Could you check a few things on this model? Use its own coordinates, in mm. A direction names the side the tool comes from. Coordinates: 2 decimals unless noted, no trailing zeros. Order: outer loops, then holes, each group sorted by start corner. A loop starts at its lowest first (then second) coordinate and runs counter-clockwise, first axis right, second up. Notation, with made-up numbers: (20, 57) -> (39, 57) arc R32 ccw to (39, 85) -> close; hole circle Ø4 at (3.5, -24). An arc over 180 degrees is marked (long way). Return JSON: item names as keys, results as strings. Group by question number.
Autodesk Inventor part; units mm, degrees
ref_plane "YZ Plane" through (0, 0, 0) normal (1, 0, 0) x (0, 1, 0)
ref_plane "XZ Plane" through (0, 0, 0) normal (0, 1, 0) x (-1, 0, 0)
ref_plane "XY Plane" through (0, 0, 0) normal (0, 0, 1) x (1, 0, 0)
sketch "Sketch1" plane through (0, 0, 0) normal (0, 1, 0) x (-1, 0, 0)
  line L0 (0, 0) -> (12, 0)
  line L1 (12, 0) -> (12, -144.6)
  line L2 (12, -144.6) -> (0, -144.6)
  line L3 (0, -144.6) -> (0, 0)
  line L4 (0, 0) -> (3, 0)
  line L5 (3, 0) -> (3, -4)
  line L6 (3, -4) -> (0, -4)
  line L7 (0, -4) -> (0, 0)
  line L8 (3, -4) -> (9, -4)
  circle A0 centre (9, -4) radius 1.5
  circle A1 centre (3, -4) radius 1.5
  line L9 (12, -144.6) -> (9, -144.6)
  line L10 (9, -144.6) -> (9, -140.6)
  line L11 (9, -140.6) -> (12, -140.6)
  line L12 (12, -140.6) -> (12, -144.6)
  line L13 (9, -140.6) -> (3, -140.6)
  circle A2 centre (9, -140.6) radius 1.5
  circle A3 centre (3, -140.6) radius 1.5
  dimension "d0" = 12
  dimension "d1" = 144.6
  dimension "d2" = 3
  dimension "d3" = 4
  dimension "d4" = 6
  dimension "d5" = 3
  dimension "d6" = 3
  dimension "d7" = 3
  dimension "d8" = 4
  dimension "d9" = 6
  dimension "d10" = 3
  dimension "d11" = 3
extrude "Extrusion1" add sketch "Sketch1" along normal blind 3 contours L0 L5 A1 L6 L3 | L0 L1 L11 A2 L10 L2 L3 L6 A1 L5 | L1 L2 L10 A2 L11
sketch "Sketch2" plane through (0, 3, 0) normal (0, 1, 0) x (1, 0, 0)
  line L0 (-12, 0) -> (0, 0)
  line L1 (-6, 0) -> (-6, 144.6) construction
  line L2 (0, 144.6) -> (-12, 144.6)
  line L3 (-4.5, 0) -> (-4.5, 144.6)
  line L4 (-7.5, 144.6) -> (-7.5, 0)
  arc A0 (-7.5, 0) -> (-4.5, 0) centre (-6, 0) ccw
  arc A1 (-4.5, 144.6) -> (-7.5, 144.6) centre (-6, 144.6) ccw
  line L5 (0, 0) -> (0, 144.6)
  line L6 (-12, 0) -> (0, 0)
  line L7 (0, 0) -> (0, 8)
  line L8 (0, 8) -> (-12, 8)
  line L9 (-12, 8) -> (-12, 0)
  line L10 (-12, 144.6) -> (0, 144.6)
  line L11 (0, 144.6) -> (0, 136.6)
  line L12 (0, 136.6) -> (-12, 136.6)
  line L13 (-12, 136.6) -> (-12, 144.6)
  point P0 (-6, 72.3)
  point P1 (-4.5, 136.6)
  point P2 (-7.5, 136.6)
  point P3 (-7.5, 8)
  point P4 (-4.5, 8)
  dimension "d14" = 3
  dimension "d15" = 8
  dimension "d16" = 8
extrude "Extrusion2" add sketch "Sketch2" along normal blind 3 contours L4 L12 L3 L8
fillet "Fillet1" radius 3 2 edges at (-6, 6, -8) (-6, 6, -136.6)
fillet "Fillet2" radius 3 4 edges at (0, 1.5, 0) (-12, 1.5, 0) (-12, 1.5, -144.6) (0, 1.5, -144.6)
fillet "Fillet3" radius 1.5 6 edges at (-7.5, 5.1215, -8.8785) (-7.5, 5.1215, -135.7215) (-7.5, 6, -72.3) (-4.5, 5.1215, -135.7215) (-4.5, 5.1215, -8.8785) (-4.5, 6, -72.3)
sketch "Sketch3" plane through (0, 3, 0) normal (0, 1, 0) x (1, 0, 0)
  line L0 (-12, 141.6) -> (-12, 3)
  line L1 (-12, 72.3) -> (-6, 72.3)
  line L2 (-9, 42.3) -> (-3, 42.3)
  line L3 (-3, 42.3) -> (-3, 102.3)
  line L4 (-3, 102.3) -> (-9, 102.3)
  line L5 (-9, 102.3) -> (-9, 42.3)
  line L6 (-9, 42.3) -> (-3, 102.3) construction
  line L7 (-3, 42.3) -> (-9, 102.3) construction
  line L8 (-9, 32.3) -> (-3, 32.3)
  line L9 (-3, 32.3) -> (-3, 112.3)
  line L10 (-3, 112.3) -> (-9, 112.3)
  line L11 (-9, 112.3) -> (-9, 32.3)
  line L12 (-9, 32.3) -> (-3, 112.3) construction
  line L13 (-3, 32.3) -> (-9, 112.3) construction
  line L14 (-9, 112.3) -> (-3, 112.3) construction
  line L15 (-9, 109.3) -> (-3, 109.3)
  line L16 (-3, 115.3) -> (-9, 115.3)
  arc A0 (-9, 115.3) -> (-9, 109.3) centre (-9, 112.3) ccw
  arc A1 (-3, 109.3) -> (-3, 115.3) centre (-3, 112.3) ccw
  circle A2 centre (-9, 112.3) radius 1.5
  circle A3 centre (-3, 112.3) radius 1.5
  circle A4 centre (-9, 102.3) radius 1.5
  circle A5 centre (-3, 102.3) radius 1.5
  line L17 (-9, 102.3) -> (-3, 102.3) construction
  line L18 (-9, 99.3) -> (-3, 99.3)
  line L19 (-3, 105.3) -> (-9, 105.3)
  arc A6 (-9, 105.3) -> (-9, 99.3) centre (-9, 102.3) ccw
  arc A7 (-3, 99.3) -> (-3, 105.3) centre (-3, 102.3) ccw
  line L20 (-3, 32.3) -> (-9, 32.3)
  line L21 (-3, 42.3) -> (-9, 42.3)
  line L22 (-9, 42.3) -> (-3, 42.3) construction
  line L23 (-9, 39.3) -> (-3, 39.3)
  line L24 (-3, 45.3) -> (-9, 45.3)
  arc A8 (-9, 45.3) -> (-9, 39.3) centre (-9, 42.3) ccw
  arc A9 (-3, 39.3) -> (-3, 45.3) centre (-3, 42.3) ccw
  circle A10 centre (-9, 42.3) radius 1.5
  circle A11 centre (-3, 42.3) radius 1.5
  circle A12 centre (-9, 32.3) radius 1.5
  circle A13 centre (-3, 32.3) radius 1.5
  line L25 (-9, 32.3) -> (-3, 32.3) construction
  line L26 (-9, 29.3) -> (-3, 29.3)
  line L27 (-3, 35.3) -> (-9, 35.3)
  arc A14 (-9, 35.3) -> (-9, 29.3) centre (-9, 32.3) ccw
  arc A15 (-3, 29.3) -> (-3, 35.3) centre (-3, 32.3) ccw
  point P0 (0, 0)
  point P1 (-6, 112.3)
  point P2 (-6, 102.3)
  point P3 (-6, 42.3)
  point P4 (-6, 32.3)
  dimension "d22" = 6
  dimension "d23" = 6
  dimension "d24" = 60
  dimension "d25" = 6
  dimension "d26" = 80
  dimension "d27" = 6
  dimension "d28" = 3
  dimension "d29" = 3
  dimension "d30" = 3
  dimension "d31" = 3
  dimension "d32" = 6
  dimension "d33" = 6
  dimension "d34" = 6
  dimension "d35" = 6
  dimension "d36" = 3
  dimension "d37" = 3
  dimension "d38" = 3
  dimension "d39" = 3
  dimension "d40" = 6
extrude "Extrusion3" cut sketch "Sketch3" along normal blind 3 contours A0 L16 A1 L9 A3 L10 A2 L11 | A6 L11 A4 L5 | L11 A2 L10 A3 L9 L15 | L19 L9 A5 L4 A4 L11 | L5 A4 L4 A5 L3 L18 | A8 L5 A10 L11 | A7 L3 A5 L9 | A14 L11 A12 L8 A13 L9 A15 L26 | L24 L3 A11 L2 A10 L5 | L11 A10 L2 A11 L9 L23 | A9 L9 A11 L3 | L27 L9 A13 L8 A12 L11
extrude "Extrusion4" cut sketch "Sketch3" against normal blind 3 contours A2 L10 L11 | L11 L10 A2 | A4 L4 L11 | L11 L5 A4 | L5 L4 A4 | A3 L10 L9 | L9 L10 A3 | A5 L3 L9 | L9 L4 A5 | A5 L4 L3 | A10 L2 L5 | L5 L11 A10 | L11 L2 A10 | A11 L9 L3 | L3 L2 A11 | A12 L8 L11 | L11 L8 A12 | A11 L2 L9 | A13 L8 L9 | L9 L8 A13
properties part number "structural_bar1"
Q1. On a 3-axis mill with a long thin cutter (end or side, diameter ignored), from which of +Z, -Z, +X, -X, +Y, -Y can I reach the whole of each face in a straight line? I mean faces 4 (the cylindrical face through (-11.14, 1.52, -0.9)), 5 (the flat face through (-6, 4, -35.3)). Say none if no direction works.
Q2. I want a section at A-A on y = 1.8. State how many separate pieces and enclosed holes the cut face has, and give its area (3 significant figures).
Q3. I'm going to push flat-ended pins straight in: pin 1 Ø1.2 at (y, z) = (4, -38.5) entering from +X; pin 2 Ø1.5 at (x, y) = (-6, 4) entering from -Z; pin 3 Ø3 at (x, z) = (-1.5, -81) entering from +Y. Where does each tip first touch, or does it pass through?
Q4. We'd pull the mould along X, two halves only. Please class faces 1 (the cylindrical face through (-11.1, 1.52, -143.74)), 2 (the cylindrical face through (-2.194, 1.521, -113.565)), 3 (the flat face through (-6, 4, -105.3)): pulls with the +X half, pulls with the -X half, needs draft (parallel to the pull), parting line crosses it, or undercut.
Q5. I need wall thicknesses on line 1 along X through (y, z) = (2.7, -102.5); line 2 along Z through (x, y) = (-6, 3.9); line 3 along X through (y, z) = (4.35, -71.5). Which ranges of each line are inside material? Lowest first, please. Write a range as from..to.
Q6. I want a section at B-B on z = -102.3. Please give me the cut outline in (x, y), and give its area (3 significant figures).
Response values:
{
 "1": {"face 4": "+Z, -X, +Y, -Y", "face 5": "+X, -X, +Y"},
 "2": {"separate pieces": "1", "enclosed holes": "12", "area": "1,640 mm²"},
 "3": {"pin 1": "stops at x = -4.5", "pin 2": "stops at z = -136.59", "pin 3": "stops at y = 3"},
 "4": {"face 1": "pulls with the -X half", "face 2": "undercut", "face 3": "needs draft"},
 "5": {"line 1": "x = -12..-10.49, -7.51..-4.49, -1.51..0", "line 2": "z = -136.46..-115.3, -109.3..-105.3, -99.3..-45.3, -39.3..-35.3, -29.3..-8.14", "line 3": "x = -7.5..-4.5"},
 "6": {"outline": "(-12, 0) -> (-10.5, 0) -> (-10.5, 3) -> (-12, 3) -> close; (-7.5, 0) -> (-4.5, 0) -> (-4.5, 3) -> (-7.5, 3) -> close; (-1.5, 0) -> (0, 0) -> (0, 3) -> (-1.5, 3) -> close", "area": "18.0 mm²"}
}
